Part model, mm, in its own coordinate system. Round coordinates to 2 decimals unless told otherwise and drop trailing zeros. Loops run counter-clockwise (first coordinate to the right, second up) from the corner with the lowest first, then second, coordinate; pieces in that order, holes last.
from build123d import *

# Parameters (mm, degrees)
SKETCH1_R           = 25
SKETCH1_R_2         = 4.5
BOSS_EXTRUDE1_DEPTH = 3
SKETCH2_R           = 1.5
CUT_EXTRUDE1_DEPTH  = 36.482389998
CIRPATTERN1_COUNT   = 4
SKETCH3_R           = 1.5
CUT_EXTRUDE3_DEPTH  = 36.482389998
CIRPATTERN2_COUNT   = 4


with BuildPart() as part:
    # Sketch1 → Boss-Extrude1 (new body)
    with BuildSketch(Plane(origin=(0, 0, 0), x_dir=(1, 0, 0), z_dir=(0, 1, 0))):
        with Locations(Location((0, 0, 0), (0, 0, 270))):
            Circle(SKETCH1_R)
        with Locations(Location((0, 0, 0), (0, 0, 270))):
            Circle(SKETCH1_R_2, mode=Mode.SUBTRACT)
    extrude(amount=BOSS_EXTRUDE1_DEPTH)

    # Sketch2 → Cut-Extrude1 (cut, through all)
    with BuildSketch(Plane(origin=(0, 3, 0), x_dir=(1, 0, 0), z_dir=(0, 1, 0))):
        with Locations(Location((0, 8.5, 0), (0, 0, 270))):
            Circle(SKETCH2_R)
    cut_extrude1 = extrude(amount=-CUT_EXTRUDE1_DEPTH, mode=Mode.SUBTRACT)

    # CirPattern1: Cut-Extrude1 ×4 about axis
    cirpattern1_axis = Axis((0, 0, 0), (0, 1, 0))
    for i in range(1, CIRPATTERN1_COUNT):
        add(cut_extrude1.rotate(cirpattern1_axis, i * 360 / CIRPATTERN1_COUNT), mode=Mode.SUBTRACT)

    # Sketch3 → Cut-Extrude3 (cut, through all)
    with BuildSketch(Plane(origin=(0, 3, 0), x_dir=(1, 0, 0), z_dir=(0, 1, 0))):
        with Locations(Location((0, 22, 0), (0, 0, 270))):
            Circle(SKETCH3_R)
    cut_extrude3 = extrude(amount=-CUT_EXTRUDE3_DEPTH, mode=Mode.SUBTRACT)

    # CirPattern2: Cut-Extrude3 ×4 about axis
    cirpattern2_axis = Axis((0, 0, 0), (0, 1, 0))
    for i in range(1, CIRPATTERN2_COUNT):
        add(cut_extrude3.rotate(cirpattern2_axis, i * 360 / CIRPATTERN2_COUNT), mode=Mode.SUBTRACT)


solid = part.part
1) Mould opens along Z. For faces 1 (the face through (-10, 2, 0)), 2 (the face through (7.509, 1.479, 23.846)), 3 (the face through (0, 3, 5)) say: released by +Z, released by -Z, zero draft, split by the parting line, or undercut.
Values:
face 1: undercut
face 2: split by the parting line
face 3: zero draft
2) Wall check: line 1 along Z through (x, y) = (-1, 1.15); line 2 along X through (y, z) = (2.1, 8.5). Give the ranges that are in metal, low to high.
Values:
line 1: z = -24.98 to -23.12, -20.88 to -9.62, -7.38 to -4.39, 4.39 to 7.38, 9.62 to 20.88, 23.12 to 24.98
line 2: x = -23.51 to -1.5, 1.5 to 23.51
3) Slice it at A-A, the plane y = 0.5. Give the number of separate pieces and of enclosed holes in the cut face, then the cut area to 3 significant figures.
Values:
separate pieces: 1
enclosed holes: 9
area: 1,840 mm2
4) Slice it at C-C, the plane z = -8.5. Give the cut face in (x, y).
Values:
outline: (-23.51, 0) - (-1.5, 0) - (-1.5, 3) - (-23.51, 3) - close; (1.5, 0) - (23.51, 0) - (23.51, 3) - (1.5, 3) - close
5) Drop flat-ended pins along their axis: pin 1 Ø1 at (y, z) = (1.5, -14.5) entering from +X; pin 2 Ø1 at (x, y) = (3.5, 1.5) entering from -Z; pin 3 Ø1 at (x, y) = (-17.5, 0.5) entering from -Z. Give the stop position or say it passes through.
Values:
pin 1: stops at x = 20.71
pin 2: stops at z = -24.82
pin 3: stops at z = -18.33
6) Slice it at D-D, the plane x = -8.5. Give the cut face in (y, z), then the cut area to 3 significant figures.
Values:
outline: (0, -23.51) - (3, -23.51) - (3, -1.5) - (0, -1.5) - close; (0, 1.5) - (3, 1.5) - (3, 23.51) - (0, 23.51) - close
area: 132 mm2
7) Slice it at B-B, the plane x = 0. Give the cut face in (y, z), then the cut area to 3 significant figures.
Values:
outline: (0, -25) - (3, -25) - (3, -23.5) - (0, -23.5) - close; (0, -20.5) - (3, -20.5) - (3, -10) - (0, -10) - close; (0, -7) - (3, -7) - (3, -4.5) - (0, -4.5) - close; (0, 4.5) - (3, 4.5) - (3, 7) - (0, 7) - close; (0, 10) - (3, 10) - (3, 20.5) - (0, 20.5) - close; (0, 23.5) - (3, 23.5) - (3, 25) - (0, 25) - close
area: 87.0 mm2
